Geometry check sheet. Reference: the model listing, model coordinates, mm. A direction names the side the tool comes from. Round coordinates to 2 decimals unless told otherwise and drop trailing zeros. Order: outer loops, then holes, each group sorted by start corner. A loop starts at its lowest first (then second) coordinate and runs counter-clockwise, first axis right, second up. Notation, with made-up numbers: (-16.5, 54.25) -> (32.5, 54.25) arc R25 cw to (32.5, 91.25) -> close; hole circle Ø5 at (27, 20). An arc over 180 degrees is marked (long way). Use a Markdown table: item, result. Add a question column.
Item 1: Material ranges on probe 1 along Z at (x, y) = (-51.25, 42.25); probe 2 along X at (y, z) = (41.25, 8.75); probe 3 along X at (y, z) = (50.75, 8.5), recorded low to high. Write a range as [from, to].
Item 2: Sectioned sample at A-A, the plane z = 4. Record the cut outline in (x, y), and give its area (3 significant figures).
Item 3: Gauge pin test, flat ends, axial feed: pin 1 Ø1 at (y, z) = (41, 3) entering from -X; pin 2 Ø4 at (x, z) = (-48, 4.5) entering from +Y (3 decimals); pin 3 Ø1 at (x, z) = (-51.5, 2.5) entering from -Y. Record the tip position at first contact, or that the pin passes through.
Item 4: Sectioned sample at C-C, the plane z = 8.25. Record the cut outline in (x, y).
Item 5: Sectioned sample at B-B, the plane y = 41.25. Record the cut outline in (x, z), and give its area (3 significant figures).
Item 6: Set-up check for faces 1 (the cylindrical face through (-38.4, 51.89, 8.17)), 2 (the flat face through (-41.84, 53.54, 4.98)): record each of +Z, -Z, +X, -X, +Y, -Y from which the full face is reachable in a straight line by a thin tool's end or side.
Item 7: Mould release check, pull along X, two halves, no side actions. Record for faces 3 (the flat face through (-53.81, 36.57, 4.93)), 4 (the flat face through (-46, 46, 7.95)), 5 (the flat face through (-44, 48, 4)): pulls with the +X half, pulls with the -X half, needs draft (parallel to the pull), parting line crosses it, or undercut.
Item 8: Sectioned sample at D-D, the plane y = 51.5. Record the cut outline in (x, z).
Autodesk Fusion 360 part; units mm, degrees
sketch "Skizze1" plane through (0, 0, 0) normal (0, 0, 1) x (1, 0, 0)
  circle A0 centre (0, 0) radius 65 construction
  line L0 (-66.7503, 52.1511) -> (89.6233, -70.0214) construction
  line L1 (-51.5684, 66.0045) -> (50.4838, -64.6164) construction
  line L2 (-86.5753, 0) -> (92.1282, 0) construction
  line L3 (0, 84.3443) -> (0, -71.5181) construction
  circle A1 centre (0, 0) radius 60.6
  circle A2 centre (0, 0) radius 69.4
  line L4 (-42.8236, 63.013) -> (41.6736, -61.3209)
  line L5 (-61.3482, 41.6922) -> (84.2724, -57.2715)
  circle A3 centre (-51.2207, 40.018) radius 1.75
  circle A4 centre (-40.018, 51.2207) radius 1.75
  line L6 (-91.6282, 91.6282) -> (70.0913, -70.0913) construction
  line L7 (-102.9597, -11.0359) -> (6.8047, 98.7286) construction
  point P0 (-51.2207, 40.018)
  point P1 (-40.018, 51.2207)
  point P2 (-51.2207, 40.018)
  point P3 (-40.018, 51.2207)
  point P4 (-45.9619, 45.9619)
  dimension "d1" = 130
  dimension "d2" = 38
  dimension "d3" = 38
  dimension "d4" = 121.2
  dimension "d5" = 138.8
  dimension "d6" = 34.2
  dimension "d7" = 34.2
  dimension "d10" = 3.5
  dimension "d11" = 3.5
  dimension "d12" = 45
ref_plane "Arbeitsebene1" through (0, 0, 0) normal (0.7071, 0.7071, 0) x (-0.7071, 0.7071, 0)
sketch "Skizze3" plane through (0, 0, 0) normal (0.7071, 0.7071, 0) x (-0.7071, 0.7071, 0)
  line L0 (65, 53.8628) -> (65, -35) construction
  point P0 (65, 0)
ref_plane "Arbeitsebene2" through (-45.9619, 45.9619, 0) normal (0.7071, -0.7071, 0) x (0.7071, 0.7071, 0)
sketch "Skizze4" plane through (-45.9619, 45.9619, 0) normal (0.7071, -0.7071, 0) x (0.7071, 0.7071, 0)
  line L0 (0, 44.1227) -> (0, -35) construction
  line L1 (53.181, 0) -> (-38.9604, 0) construction
  line L2 (51.233, 5) -> (-51.6226, 5) construction
  line L3 (1.7032, 2.05) -> (3.4064, 5)
  line L4 (3.4064, 5) -> (1.7032, 7.95)
  line L5 (1.7032, 7.95) -> (-1.7032, 7.95)
  line L6 (-1.7032, 7.95) -> (-3.4064, 5)
  line L7 (-3.4064, 5) -> (-1.7032, 2.05)
  line L8 (-1.7032, 2.05) -> (1.7032, 2.05)
  line L9 (3.4064, 7.95) -> (-3.4064, 7.95)
  line L10 (-3.4064, 7.95) -> (-3.4064, 5)
  line L11 (-3.4064, 5) -> (3.4064, 5)
  line L12 (3.4064, 5) -> (3.4064, 7.95)
  circle A0 centre (0, 5) radius 1.75
  point P0 (0, 5)
  dimension "d13" = 5
  dimension "d15" = 5.9
  dimension "d28" = 3.5
extrude "Extrusion1" add sketch "Skizze1" along normal blind 10 contours A1 A2 L4 L5 picked at (-47.8032, 46.0094)
extrude "Extrusion2" cut sketch "Skizze4" along normal mid plane 2.8
ref_plane "Arbeitsebene3" through (0, 0, 5) normal (0, 0, 1) x (1, 0, 0)
sketch "Skizze5" plane through (0, 0, 5) normal (0, 0, 1) x (1, 0, 0)
  line L0 (-43.0431, 55.0926) -> (33.9956, -43.5124) construction
  line L1 (-63.2817, 49.4411) -> (43.7853, -34.2088) construction
  line L2 (-70, 0) -> (67.6704, 0) construction
  line L3 (0, 69.2816) -> (0, -27.82) construction
  circle A0 centre (0, 0) radius 65 construction
  line L4 (-36.8485, 49.9727) -> (-37.3524, 53.3415)
  line L5 (-37.3524, 53.3415) -> (-40.5219, 54.5896)
  line L6 (-40.5219, 54.5896) -> (-43.1875, 52.4687)
  line L7 (-43.1875, 52.4687) -> (-42.6836, 49.0999)
  line L8 (-42.6836, 49.0999) -> (-39.5141, 47.8518)
  line L9 (-39.5141, 47.8518) -> (-36.8485, 49.9727)
  line L10 (-47.8518, 39.5141) -> (-49.0999, 42.6836)
  line L11 (-49.0999, 42.6836) -> (-52.4687, 43.1875)
  line L12 (-52.4687, 43.1875) -> (-54.5896, 40.5219)
  line L13 (-54.5896, 40.5219) -> (-53.3415, 37.3524)
  line L14 (-53.3415, 37.3524) -> (-49.9727, 36.8485)
  line L15 (-49.9727, 36.8485) -> (-47.8518, 39.5141)
  point P0 (-40.018, 51.2207)
  point P1 (-51.2207, 40.018)
  point P2 (-40.018, 51.2207)
  point P3 (-51.2207, 40.018)
  dimension "d21" = 38
  dimension "d22" = 38
  dimension "d23" = 130
  dimension "d24" = 5.9
  dimension "d25" = 5.9
extrude "Extrusion3" cut sketch "Skizze5" along normal mid plane 2.8
extrude "Extrusion4" cut sketch "Skizze4" along normal mid plane 30 contours L11 A0 | L11 A0
Found:
| question | item | result |
|---|---|---|
| 1 | probe 1 | z = [0, 3.6], [6.4, 10] |
| 1 | probe 2 | x = [-55.81, -52.46], [-49.98, -44.39] |
| 1 | probe 3 | x = [-47.34, -41.7], [-38.33, -34.49] |
| 2 | outline | (-57.4, 39.01) -> (-50.12, 34.06) arc R60.6 cw to (-43.85, 41.82) -> (-45.99, 43.96) -> (-46.97, 42.97) -> (-48.95, 44.95) -> (-47.97, 45.94) -> (-50.08, 48.05) arc R69.4 ccw to start; (-48.05, 50.08) -> (-45.94, 47.97) -> (-44.95, 48.95) -> (-42.97, 46.97) -> (-43.96, 45.99) -> (-41.82, 43.85) arc R60.6 cw to (-34.06, 50.12) -> (-39.01, 57.4) arc R69.4 ccw to start; hole (-54.59, 40.52) -> (-53.34, 37.35) -> (-49.97, 36.85) -> (-47.85, 39.51) -> (-49.1, 42.68) -> (-52.47, 43.19) -> close; hole (-43.19, 52.47) -> (-42.68, 49.1) -> (-39.51, 47.85) -> (-36.85, 49.97) -> (-37.35, 53.34) -> (-40.52, 54.59) -> close |
| 2 | area | 122 mm2 |
| 3 | pin 1 | stops at x = -56.36 |
| 3 | pin 2 | stops at y = 51.965 |
| 3 | pin 3 | stops at y = 34.66 |
| 4 | outline | (-57.4, 39.01) -> (-50.12, 34.06) arc R60.6 cw to (-34.06, 50.12) -> (-39.01, 57.4) arc R69.4 ccw to start; hole circle Ø3.5 at (-51.22, 40.02); hole circle Ø3.5 at (-40.02, 51.22) |
| 5 | outline | (-55.81, 0) -> (-52.46, 0) -> (-52.46, 3.6) -> (-54.01, 3.6) -> (-54.01, 6.4) -> (-52.46, 6.4) -> (-52.46, 10) -> (-55.81, 10) -> close; (-49.98, 0) -> (-44.39, 0) -> (-44.39, 10) -> (-49.98, 10) -> (-49.98, 6.4) -> (-48.54, 6.4) -> (-48.54, 3.6) -> (-49.98, 3.6) -> close |
| 5 | area | 80.9 mm2 |
| 6 | face 1 | +Z, -Z |
| 6 | face 2 | none |
| 7 | face 3 | pulls with the -X half |
| 7 | face 4 | undercut |
| 7 | face 5 | undercut |
| 8 | outline | (-46.52, 0) -> (-41.75, 0) -> (-41.75, 3.6) -> (-43.04, 3.6) -> (-43.04, 6.4) -> (-41.75, 6.4) -> (-41.75, 10) -> (-46.52, 10) -> close; (-38.29, 0) -> (-35, 0) -> (-35, 10) -> (-38.29, 10) -> (-38.29, 6.4) -> (-37.08, 6.4) -> (-37.08, 3.6) -> (-38.29, 3.6) -> close |
